Geometry: final body of the model. Coordinates: model frame, mm. Face numbers are marked on the shaded views. A direction names the side the tool comes from. Coordinates: 2 decimals unless noted, no trailing zeros. Order: outer loops, then holes, each group sorted by start corner. A loop starts at its lowest first (then second) coordinate and runs counter-clockwise, first axis right, second up. Notation, with made-up numbers: M 9,73.5 L 14,73.5 A11 cw 14,89.5 Z; hole C 34,27 d7. An arc over 180 degrees is marked long. One line per question, with ' | ' between items.
from build123d import *

# Parameters (mm, degrees)
SKETCH_1_W          = 65
SKETCH_1_H          = 11
EXTRUDE_1_DEPTH     = 20
EXTRUDE_1_2_DEPTH   = 20
SKETCH_2_W          = 65
SKETCH_2_H          = 42
EXTRUDE_2_DEPTH     = 5
SKETCH_3_W          = 5
SKETCH_3_H          = 42
EXTRUDE_3_DEPTH     = 42
SKETCH_5_R          = 12
SKETCH_5_R_2        = 3
CUT_EXTRUDE_3_DEPTH = 42


with BuildPart() as part:
    # Sketch 1 → Extrude 1 (new body)
    with BuildSketch(Plane(origin=(0, 0, 0), x_dir=(1, 0, 0), z_dir=(0, 1, 0))):
        with Locations((8.014018692, 3.47352182)):
            Rectangle(SKETCH_1_W, SKETCH_1_H)
    extrude(amount=EXTRUDE_1_DEPTH)



with BuildPart() as body_2:
    # Sketch 1 → Extrude 1 2 (new body)
    with BuildSketch(Plane(origin=(0, 0, 0), x_dir=(1, 0, 0), z_dir=(0, 1, 0))):
        with Locations((8.014018692, -27.52647818)):
            Rectangle(SKETCH_1_W, SKETCH_1_H)
    extrude(amount=EXTRUDE_1_2_DEPTH)


with BuildPart() as part_1:
    add(part.part)

    add(body_2.part)  # Extrude 2 merges body 2
    # Sketch 2 → Extrude 2 (add)
    with BuildSketch(Plane(origin=(0, 20, 0), x_dir=(1, 0, 0), z_dir=(0, 1, 0))):
        with Locations((8.014018692, -12.02647818)):
            Rectangle(SKETCH_2_W, SKETCH_2_H)
    extrude(amount=EXTRUDE_2_DEPTH)

    # Sketch 3 → Extrude 3 (add)
    with BuildSketch(Plane(origin=(0, 25, 0), x_dir=(1, 0, 0), z_dir=(0, 1, 0))):
        with Locations((-21.985981308, -12.02647818)):
            Rectangle(SKETCH_3_W, SKETCH_3_H)
    extrude(amount=EXTRUDE_3_DEPTH)

    # Sketch 5 → Cut-Extrude 3 (cut)
    with BuildSketch(Plane(origin=(-19.485981308, 0, 0), x_dir=(0, 0, -1), z_dir=(1, 0, 0))):
        with Locations((-12.02647818, 46)):
            Circle(SKETCH_5_R)
        with Locations((-28.02647818, 62)):
            Circle(SKETCH_5_R_2)
        with Locations((3.97352182, 62)):
            Circle(SKETCH_5_R_2)
        with Locations((3.97352182, 30)):
            Circle(SKETCH_5_R_2)
        with Locations((-28.02647818, 30)):
            Circle(SKETCH_5_R_2)
    extrude(amount=-CUT_EXTRUDE_3_DEPTH, mode=Mode.SUBTRACT)


solid = part_1.part
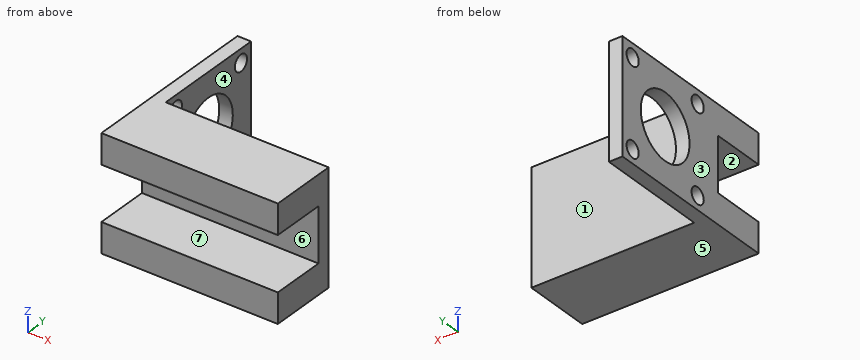
1. Section C-C, the plane z = 28.5. Output: boundary loops of the cut face in (x, y), and give its area (3 significant figures).
Response values:
outline: M -24.49,0 L 40.51,0 L 40.51,25 L -19.49,25 L -19.49,27.04 L -24.49,27.04 Z; M -24.49,32.96 L -19.49,32.96 L -19.49,59.04 L -24.49,59.04 Z; M -24.49,64.96 L -19.49,64.96 L -19.49,67 L -24.49,67 Z | area: 1,780 mm^2
2. Section B-B, the plane y = 46. Output: boundary loops of the cut face in (x, z), and give its area (3 significant figures).
Response values:
outline: M -24.49,-8.97 L -19.49,-8.97 L -19.49,0.03 L -24.49,0.03 Z; M -24.49,24.03 L -19.49,24.03 L -19.49,33.03 L -24.49,33.03 Z | area: 90.0 mm^2
3. Material intervals for line 1 (Z direction, x = 27.5, y = 16.5); line 2 (Y direction, x = 16.5, z = 23); line 3 (X direction, y = 54, z = 31), sorted ascending. Write a range as [from, to].
Response values:
line 1: z = [-8.97, 2.03], [22.03, 33.03] | line 2: y = [0, 25] | line 3: x = [-24.49, -19.49]
4. Section D-D, the plane x = 30. Output: boundary loops of the cut face in (y, z).
Response values:
outline: M 0,-8.97 L 25,-8.97 L 25,33.03 L 0,33.03 L 0,22.03 L 20,22.03 L 20,2.03 L 0,2.03 Z
5. Section A-A, the plane y = 30. Output: boundary loops of the cut face in (x, z), and give its area (3 significant figures).
Response values:
outline: M -24.49,-8.97 L -19.49,-8.97 L -19.49,-6.97 L -24.49,-6.97 Z; M -24.49,-0.97 L -19.49,-0.97 L -19.49,25.03 L -24.49,25.03 Z; M -24.49,31.03 L -19.49,31.03 L -19.49,33.03 L -24.49,33.03 Z | area: 150 mm^2
6. Access query for the marked faces 1, 2 and 3. Directions: +Z, -Z, +X, -X, +Y, -Y. A direction counts if a zero-diameter tool reaches every point of the face in a straight line with its end or side. Return the directions, or none.
Response values:
face 1: +Z, -Z, +X, +Y | face 2: +X, -X, -Y | face 3: +Z, -Z, -X, +Y, -Y
7. Draft query along Z for the marked faces 4, 5, 6 and 7. Return one class per face: pulls with the +Z half, pulls with the -Z half, needs draft (parallel to the pull), parting line crosses it, or undercut.
Response values:
face 4: needs draft | face 5: pulls with the -Z half | face 6: undercut | face 7: undercut
8. Pin query (flat end, axial travel): P1, Ø1, axis at x = -2, z = 17, coming from the +Y side; P2, Ø12.5, axis at y = 46.5, z = 19.5, coming from the +X side; P3, Ø5, axis at x = 9.5, z = 5.5, coming from the -Y side. Return the tip coordinate at first contact, or that it passes through.
Response values:
P1: stops at y = 25 | P2: stops at x = -19.49 | P3: stops at y = 20
